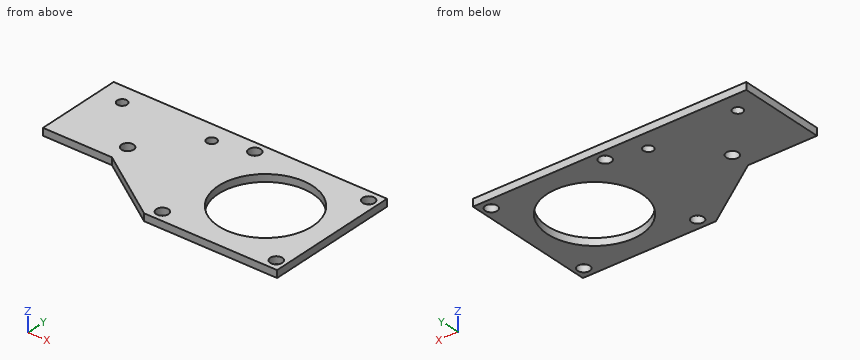
```python
from build123d import *

# Parameters (mm, degrees)
SKETCH1_W           = 113
SKETCH1_H           = 56
SKETCH1_R           = 2.5
BOSS_EXTRUDE1_DEPTH = 3
CUT_EXTRUDE1_DEPTH  = 3
SKETCH3_R           = 2.05
CUT_EXTRUDE2_DEPTH  = 10
SKETCH5_R           = 19.5
SKETCH5_R_2         = 2.5
CUT_EXTRUDE4_DEPTH  = 10


with BuildPart() as part:
    # Sketch1 → Boss-Extrude1 (new body)
    with BuildSketch(Plane.XY):
        with Locations((56.5, 28)):
            Rectangle(SKETCH1_W, SKETCH1_H)
        with Locations((28.5, 28)):
            Circle(SKETCH1_R, mode=Mode.SUBTRACT)
    extrude(amount=BOSS_EXTRUDE1_DEPTH)

    # Sketch2 → Cut-Extrude1 (cut)
    with BuildSketch(Plane.XY.offset(3)):
        Polygon((58, 0), (28.5, 20), (0, 20), (0, 28), (-30.035464335, 6.528850882), (11.479915888, -13.732243772), align=None)
    extrude(amount=-CUT_EXTRUDE1_DEPTH, mode=Mode.SUBTRACT)

    # Sketch3 → Cut-Extrude2 (cut)
    with BuildSketch(Plane(origin=(0, 0, 0), x_dir=(-1, 0, 0), z_dir=(0, 0, -1))):
        with Locations((-47.001204436, 47.999419281)):
            Circle(SKETCH3_R)
        with Locations((-10.001204503, 48.001647488)):
            Circle(SKETCH3_R)
    extrude(amount=-CUT_EXTRUDE2_DEPTH, mode=Mode.SUBTRACT)

    # Sketch5 → Cut-Extrude4 (cut)
    with BuildSketch(Plane.XY.offset(3)):
        with Locations((85.499999929, 27.997100776)):
            Circle(SKETCH5_R)
        with Locations((109.039999656, 51.534265429)):
            Circle(SKETCH5_R_2)
        with Locations((61.962835275, 51.537100503)):
            Circle(SKETCH5_R_2)
        with Locations((109.037164582, 4.457101048)):
            Circle(SKETCH5_R_2)
        with Locations((61.960000201, 4.459936122)):
            Circle(SKETCH5_R_2)
    extrude(amount=-CUT_EXTRUDE4_DEPTH, mode=Mode.SUBTRACT)


solid = part.part
```
Verification items for the finished model (mm, model axes). Coordinates: 2 decimals unless noted, no trailing zeros. Loops run counter-clockwise (first coordinate to the right, second up) from the corner with the lowest first, then second, coordinate; pieces in that order, holes last. Notation, with made-up numbers: (-3, 9) -> (12, 9) arc R27 cw to (12, 26) -> close; hole circle Ø4 at (-4, 35). An arc over 180 degrees is marked (long way). Answer in a Markdown table with one row per item. Add a question column.
1. Section check D-D, the plane z = 2.55. Give the number of separate pieces and of enclosed holes in the cut face, then the cut area to 3 significant figures.
2. Material ranges on probe 1 along Y at (x, z) = (61.96, 2.25); probe 2 along Y at (x, z) = (28.5, 1.1); probe 3 along X at (y, z) = (6.5, 1), recorded low to high. Write a range as [from, to].
3. Section check C-C, the plane x = 85.5. Enter the section's corners in (y, z).
4. Depth check by flat-ended pin: P1, Ø1.5, axis at x = 12, z = 1, coming from the -Y side. Enter the tip coordinate at first touch or a pass-through.
5. Section check B-B, the plane y = 18. Enter the section's corners in (x, z), then the cut area to 3 significant figures.
6. Section check A-A, the plane x = 109.04. Enter the section's corners in (y, z).
Derived:
| question | item | result |
|---|---|---|
| 1 | separate pieces | 1 |
| 1 | enclosed holes | 8 |
| 1 | area | 4,140 mm² |
| 2 | probe 1 | y = [0, 1.96], [6.96, 49.04], [54.04, 56] |
| 2 | probe 2 | y = [20, 25.5], [30.5, 56] |
| 2 | probe 3 | x = [48.41, 60.51], [63.41, 107.6], [110.48, 113] |
| 3 | outline | (0, 0) -> (8.5, 0) -> (8.5, 3) -> (0, 3) -> close; (47.5, 0) -> (56, 0) -> (56, 3) -> (47.5, 3) -> close |
| 4 | P1 | stops at y = 20 |
| 5 | outline | (31.45, 0) -> (68.76, 0) -> (68.76, 3) -> (31.45, 3) -> close; (102.24, 0) -> (113, 0) -> (113, 3) -> (102.24, 3) -> close |
| 5 | area | 144 mm² |
| 6 | outline | (0, 0) -> (1.96, 0) -> (1.96, 3) -> (0, 3) -> close; (6.96, 0) -> (49.03, 0) -> (49.03, 3) -> (6.96, 3) -> close; (54.03, 0) -> (56, 0) -> (56, 3) -> (54.03, 3) -> close |
